Answer from the drawing. Dimensions are ordinates in mm from the lowest x, y and z of the part. Coordinates: 2 decimals unless noted, no trailing zeros. Order: outer loops, then holes, each group sorted by start corner. A loop starts at its lowest first (then second) coordinate and runs counter-clockwise, first axis right, second up. Notation, with made-up numbers: M 22.25,60.5 L 75.25,60.5 A31 cw 75.25,97.5 Z; hole C -21.5,4.5 d10. An arc over 180 degrees is marked long. One line per question, with ' | ' between items. Start each with the question number.
1) Consider probe 1 along X at (y, z) = (45.5, 1.85); probe 2 along Y at (x, z) = (37, 2.45); probe 3 along X at (y, z) = (3.5, 3.55). Determine where each line is inside the solid, lowest interval first.
2) Find section A-A, the plane y = 53. Write down the section's boundary in (x, z).
3) Find section C-C, the plane x = 71. Write down the section's boundary in (y, z).
4) Given P1, Ø2, axis at x = 42, z = 3, coming from the +Y side, flat-ended and moving along its own axis, determine where the tip first touches the part or whether it passes through.
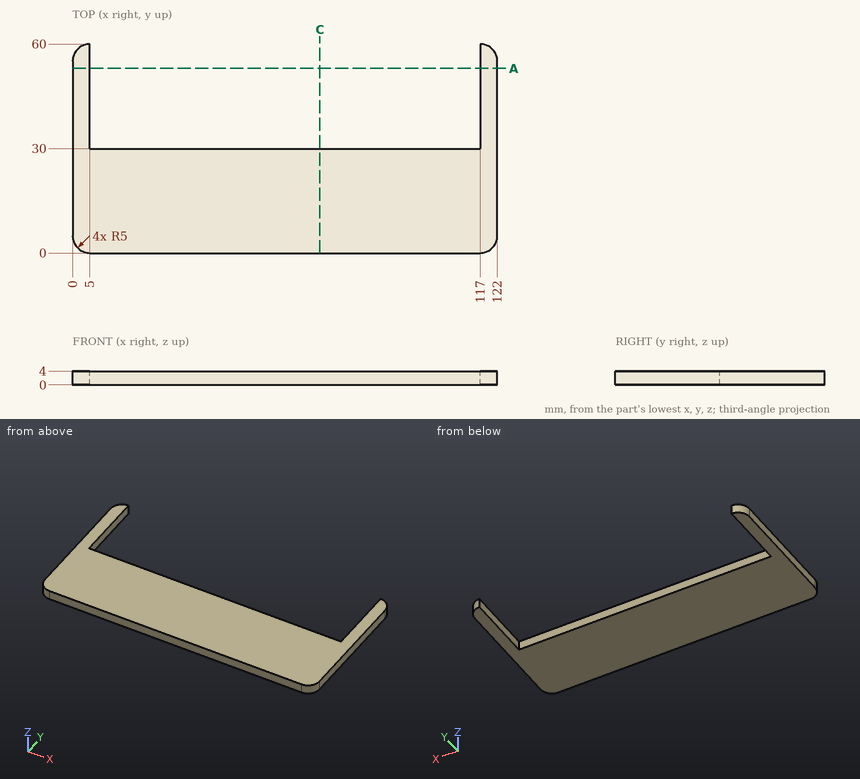
Report:
1) probe 1: x = 0 to 5, 117 to 122 | probe 2: y = 0 to 30 | probe 3: x = 0.23 to 121.77
2) outline: M 0,0 L 5,0 L 5,4 L 0,4 Z; M 117,0 L 122,0 L 122,4 L 117,4 Z
3) outline: M 0,0 L 30,0 L 30,4 L 0,4 Z
4) P1: stops at y = 30
